```python
from build123d import *

# Parameters (mm, degrees)
SKETCH1_R           = 32
SKETCH1_R_2         = 67.5
SKETCH1_W           = 36
SKETCH1_H           = 360
SKETCH1_W_2         = 360
SKETCH1_H_2         = 36
BOSS_EXTRUDE1_DEPTH = 4
SKETCH2_R           = 16
BOSS_EXTRUDE2_DEPTH = 24
SKETCH3_R           = 19
BOSS_EXTRUDE3_DEPTH = 6
CUT_EXTRUDE1_DEPTH  = 8


with BuildPart() as part:
    # Sketch1 → Boss-Extrude1 (new, symmetric)
    with BuildSketch(Plane(origin=(0, 0, 0), x_dir=(1, 0, 0), z_dir=(0, 1, 0))):
        with Locations((0, 180)):
            Circle(SKETCH1_R)
        with Locations((180, 0)):
            Circle(SKETCH1_R)
        with Locations((0, -180)):
            Circle(SKETCH1_R)
        with Locations((-180, 0)):
            Circle(SKETCH1_R)
        Circle(SKETCH1_R_2)
        Rectangle(SKETCH1_W, SKETCH1_H)
        Rectangle(SKETCH1_W_2, SKETCH1_H_2)
    extrude(amount=BOSS_EXTRUDE1_DEPTH, both=True)

    # Sketch2 → Boss-Extrude2 (add)
    with BuildSketch(Plane(origin=(0, -4, 0), x_dir=(1, 0, 0), z_dir=(0, 1, 0))):
        with Locations(Location((-180, 0, 0), (0, 0, 270))):
            Circle(SKETCH2_R)
        with Locations(Location((0, -180, 0), (0, 0, 270))):
            Circle(SKETCH2_R)
        with Locations(Location((180, 0, 0), (0, 0, 270))):
            Circle(SKETCH2_R)
        with Locations(Location((0, 180, 0), (0, 0, 270))):
            Circle(SKETCH2_R)
    extrude(amount=-BOSS_EXTRUDE2_DEPTH)

    # Sketch3 → Boss-Extrude3 (add)
    with BuildSketch(Plane(origin=(0, 4, 0), x_dir=(1, 0, 0), z_dir=(0, 1, 0))):
        with Locations(Location((-180, 0, 0), (0, 0, 270))):
            Circle(SKETCH3_R)
        with Locations(Location((0, 180, 0), (0, 0, 270))):
            Circle(SKETCH3_R)
        with Locations(Location((180, 0, 0), (0, 0, 270))):
            Circle(SKETCH3_R)
        with Locations(Location((0, -180, 0), (0, 0, 270))):
            Circle(SKETCH3_R)
    extrude(amount=BOSS_EXTRUDE3_DEPTH)

    # Sketch4 → Cut-Extrude1 (cut)
    with BuildSketch(Plane(origin=(0, 4, 0), x_dir=(1, 0, 0), z_dir=(0, 1, 0))):
        with BuildLine():
            ThreePointArc((11, 0), (-9.208416632, 6.017064329), (4.417261248, -10.074115498))
            Line((4.417261248, -10.074115498), (10.074115498, -4.417261248))
            ThreePointArc((10.074115498, -4.417261248), (10.766040834, -2.256626855), (11, 0))
        make_face()
        with BuildLine():
            Line((10.074115498, -4.417261248), (4.417261248, -10.074115498))
            ThreePointArc((4.417261248, -10.074115498), (7.778174593, -7.778174593), (10.074115498, -4.417261248))
        make_face()
        with BuildLine():
            ThreePointArc((10.074115498, -4.417261248), (7.778174593, -7.778174593), (4.417261248, -10.074115498))
            Line((4.417261248, -10.074115498), (7.283199846, -12.940054096))
            Line((7.283199846, -12.940054096), (12.940054096, -7.283199846))
            Line((12.940054096, -7.283199846), (10.074115498, -4.417261248))
        make_face()
    extrude(amount=-CUT_EXTRUDE1_DEPTH, mode=Mode.SUBTRACT)


solid = part.part
```
Check sheet for the modelled part. Datum: model origin and axes. Units: mm. A direction names the side the tool comes from. Round coordinates to 2 decimals unless told otherwise and drop trailing zeros. Loops run counter-clockwise (first coordinate to the right, second up) from the corner with the lowest first, then second, coordinate; pieces in that order, holes last. Notation, with made-up numbers: M 35,-12.5 L 67,-12.5 A13 cw 67,9.5 Z; hole C 79,-24.5 d1. An arc over 180 degrees is marked long. Answer as a JSON object with one key per item and string values.
1. Section check D-D (z = 99.5). Record the boundary of the cut face in (x, y), plus the area to 3 significant figures.
Reply:
{"outline": "M -18,-4 L 18,-4 L 18,4 L -18,4 Z", "area": "288 mm²"}
2. Section check B-B (y = -12). Record the boundary of the cut face in (x, z), plus the area to 3 significant figures.
Reply:
{"outline": "C -180,0 d32; C 0,-180 d32; C 0,180 d32; C 180,0 d32", "area": "3,220 mm²"}
3. Access from +Z, -Z, +X, -X, +Y, -Y to the whole of each face (thin tool, end or side, straight path). Record for faces 1 (the cylindrical face through (-161.16, 6.96, -2.47)), 2 (the cylindrical face through (47.384, 0.056, 48.073)), 3 (the flat face through (0, 10, -180)), 4 (the cylindrical face through (-9.736, -15.832, 167.303)), 5 (the flat face through (0, -28, 180)).
Reply:
{"face 1": "+Y", "face 2": "+Y, -Y", "face 3": "+Z, -Z, +X, -X, +Y", "face 4": "-Y", "face 5": "+Z, -Z, +X, -X, -Y"}
4. Mould release check, pull along Z, two halves, no side actions. Record for faces 6 (the flat face through (-1, -4, 15)), 7 (the flat face through (-17, 4, -1)), 8 (the cylindrical face through (170.264, -15.832, -12.697)), 9 (the flat face through (180, 10, 0)): pulls with the +Z half, pulls with the -Z half, needs draft (parallel to the pull), parting line crosses it, or undercut.
Reply:
{"face 6": "undercut", "face 7": "undercut", "face 8": "parting line crosses it", "face 9": "needs draft"}
5. Section check C-C (x = -180). Record the boundary of the cut face in (y, z).
Reply:
{"outline": "M -28,-16 L -4,-16 L -4,-32 L 4,-32 L 4,-19 L 10,-19 L 10,19 L 4,19 L 4,32 L -4,32 L -4,16 L -28,16 Z"}
6. Scan lines: line 1 (X direction, y = 0, z = 0); line 2 (Z direction, x = -123.5, y = -1.5); line 3 (Y direction, x = 132.5, z = 17). Record each from-to range of solid material in increasing order.
Reply:
{"line 1": "x = -212 to -11, 11 to 212", "line 2": "z = -18 to 18", "line 3": "y = -4 to 4"}
7. Section check A-A (z = 180). Record the boundary of the cut face in (x, y).
Reply:
{"outline": "M -32,-4 L -16,-4 L -16,-28 L 16,-28 L 16,-4 L 32,-4 L 32,4 L 19,4 L 19,10 L -19,10 L -19,4 L -32,4 Z"}
8. Gauge pin test, flat ends, axial feed: P1, Ø9, axis at x = 98, y = 1, coming from the -Z side; P2, Ø6.5, axis at y = -0.5, z = 100.5, coming from the +X side; P3, Ø1, axis at x = 30, z = 14, coming from the -Y side. Record the tip position at first contact, or that the pin passes through.
Reply:
{"P1": "stops at z = -18", "P2": "stops at x = 18", "P3": "stops at y = -4"}
